Read the model definition and answer for the solid it produces. Units are mm, in the model's axes. Round coordinates to 2 decimals unless told otherwise and drop trailing zeros. Write each loop counter-clockwise with the first axis right and the second up, starting at its lowest first coordinate (ties: lowest second). Pieces come first, ordered by that corner, then holes. Notation, with made-up numbers: (-7.5, 44) -> (41.5, 44) arc R24 ccw to (41.5, 76) -> close; hole circle Ø4 at (-28.75, -22). An arc over 180 degrees is marked (long way). Return JSON: item names as keys, results as strings. Group by question number.
(1) Straight lines are drawn through the part: line 1 (X direction, y = -115, z = 32.5); line 2 (X direction, y = -67.5, z = 21.5); line 3 (Y direction, x = 35.5, z = 31). For each, find the intervals that lie inside material, in ascending order.
(2) A cutting plane is placed at B-B on z = 3. Give the vertices of the cut face in (x, y), then the cut area to 3 significant figures.
(3) A cutting plane is placed at A-A on y = -69. Give the vertices of the cut face in (x, z), then the cut area to 3 significant figures.
(4) A cutting plane is placed at C-C on x = 43.5. Give the vertices of the cut face in (y, z).
(5) Given pin 1 (1 mm diameter, centred on y = -95, z = 21, fed in from -X); pin 2 (5 mm diameter, centred on x = 68, y = -64, fed in from +Z); pin 3 (10 mm diameter, centred on y = -82.5, z = 15.5, fed in from -X); pin 4 (6 mm diameter, centred on y = -66, z = 27, fed in from +X), each flat-ended and moving along its own axis, determine where each tip first touches the part or whether it passes through.
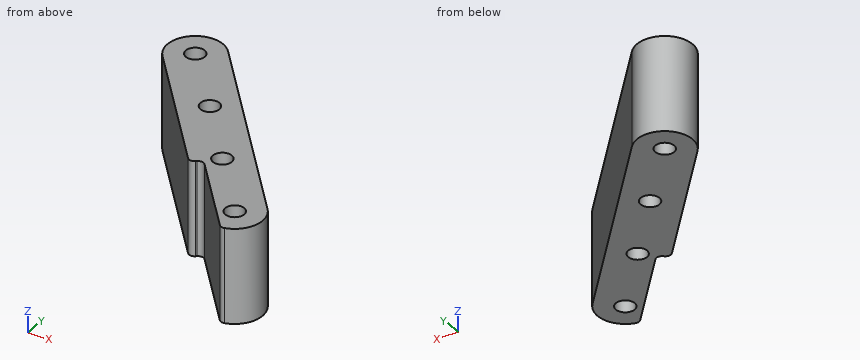
```python
from build123d import *

# Parameters (mm, degrees)
SKETCH_1_R          = 3.4
EXTRUDE_3_DEPTH     = 34
CUT_EXTRUDE_1_DEPTH = 164.659924305
FILLET_1_R          = 2


with BuildPart() as part:
    # 草图1 → 凸台-拉伸3 (new body)
    with BuildSketch(Plane.XY):
        with BuildLine():
            Line((41.331697392, -38.327914958), (99.709351413, -106.819410926))
            ThreePointArc((99.709351413, -106.819410926), (98.585524286, -120.916822482), (84.48811273, -119.792995355))
            Line((84.48811273, -119.792995355), (26.110458709, -51.301499387))
            ThreePointArc((26.110458709, -51.301499387), (27.234285836, -37.204087831), (41.331697392, -38.327914958))
        make_face()
        with Locations((33.721078051, -44.814707172)):
            Circle(SKETCH_1_R, mode=Mode.SUBTRACT)
        with Locations((53.53147549, -67.343536554)):
            Circle(SKETCH_1_R, mode=Mode.SUBTRACT)
        with Locations((72.815103781, -90.324869847)):
            Circle(SKETCH_1_R, mode=Mode.SUBTRACT)
        with Locations((92.098732071, -113.306203141)):
            Circle(SKETCH_1_R, mode=Mode.SUBTRACT)
    extrude(amount=EXTRUDE_3_DEPTH)

    # 草图2 → 切除-拉伸1 (cut, through all)
    with BuildSketch(Plane.XY.offset(34)):
        with BuildLine():
            ThreePointArc((84.48811273, -119.792995355), (88.47574874, -122.626824996), (93.330431012, -123.230059131))
            Line((93.330431012, -123.230059131), (68.680620596, -94.309705633))
            Line((68.680620596, -94.309705633), (65.255841892, -97.228762129))
            Line((65.255841892, -97.228762129), (84.48811273, -119.792995355))
        make_face()
    extrude(amount=-CUT_EXTRUDE_1_DEPTH, mode=Mode.SUBTRACT)

    # 圆角1
    fillet_1_edges = [part.edges().sort_by_distance(p)[0] for p in [
        (68.680620596, -94.309705633, 17),
        (93.330431012, -123.230059131, 17),
        (65.255841892, -97.228762129, 17),
    ]]
    fillet(fillet_1_edges, radius=FILLET_1_R)


solid = part.part
```
Checks:
{
 "1": {"line 1": "x = 86.32 to 89.15, 95.05 to 101.95", "line 2": "x = 39.92 to 50.14, 56.93 to 66.2", "line 3": "y = -62.32 to -47.71, -41.92 to -34.97"},
 "2": {"outline": "(26.11, -51.3) -> (63.96, -95.71) arc R2 ccw to (66.78, -95.93) -> (67.16, -95.61) arc R2 cw to (69.98, -95.83) -> (92.58, -122.35) arc R2 ccw to (94.6, -122.99) arc R10 ccw to (99.71, -106.82) -> (41.33, -38.33) arc R10 ccw to start; hole circle Ø6.8 at (33.72, -44.81); hole circle Ø6.8 at (53.53, -67.34); hole circle Ø6.8 at (72.82, -90.32); hole circle Ø6.8 at (92.1, -113.31)", "area": "1,810 mm^2"},
 "3": {"outline": "(41.2, 0) -> (50.56, 0) -> (50.56, 34) -> (41.2, 34) -> close; (56.5, 0) -> (67.47, 0) -> (67.47, 34) -> (56.5, 34) -> close", "area": "692 mm^2"},
 "4": {"outline": "(-71.7, 0) -> (-40.87, 0) -> (-40.87, 34) -> (-71.7, 34) -> close"},
 "5": {"pin 1": "stops at x = 62.93", "pin 2": "passes through", "pin 3": "stops at x = 48.44", "pin 4": "stops at x = 67.47"}
}
